For this review, use the dimensioned drawing (mm, ordinates from the lowest corner) and the shaded views. Round coordinates to 2 decimals unless told otherwise and drop trailing zeros. Order: outer loops, then holes, each group sorted by start corner. A loop starts at its lowest first (then second) coordinate and runs counter-clockwise, first axis right, second up. Notation, with made-up numbers: (-29.5, 59) - (4.5, 59) arc R16 cw to (4.5, 70) - close; hole circle Ø6 at (14, -30). An arc over 180 degrees is marked (long way). Write each question's results on one line, items separated by ' | '. Start each with the question number.
(1) Insertion check: pin 1 Ø6 at (x, y) = (13, 81) entering from +Z; pin 2 Ø2 at (x, z) = (41, 4.5) entering from -Y; pin 3 Ø1.9 at (y, z) = (50, 2) entering from +X; pin 4 Ø3 at (y, z) = (67.5, 3) entering from -X. Each pin has a flat end and moves straight along its axis. Give the tip position at first contact, or say it passes through.
(2) For L1, parallel to X at y = 79.5, z = 5; L2, parallel to Y at x = 13, z = 5.75, list the stretches that pass through material, from the lowest coordinate up. Write a range as from..to.
(3) Take a section at A-A, the plane z = 4. Give the boundary of the cut face in (x, y).
(4) Take a section at B-B, the plane x = 7. Give the boundary of the cut face in (y, z).
(5) Take a section at C-C, the plane y = 64.5. Give the boundary of the cut face in (x, z), plus the area to 3 significant figures.
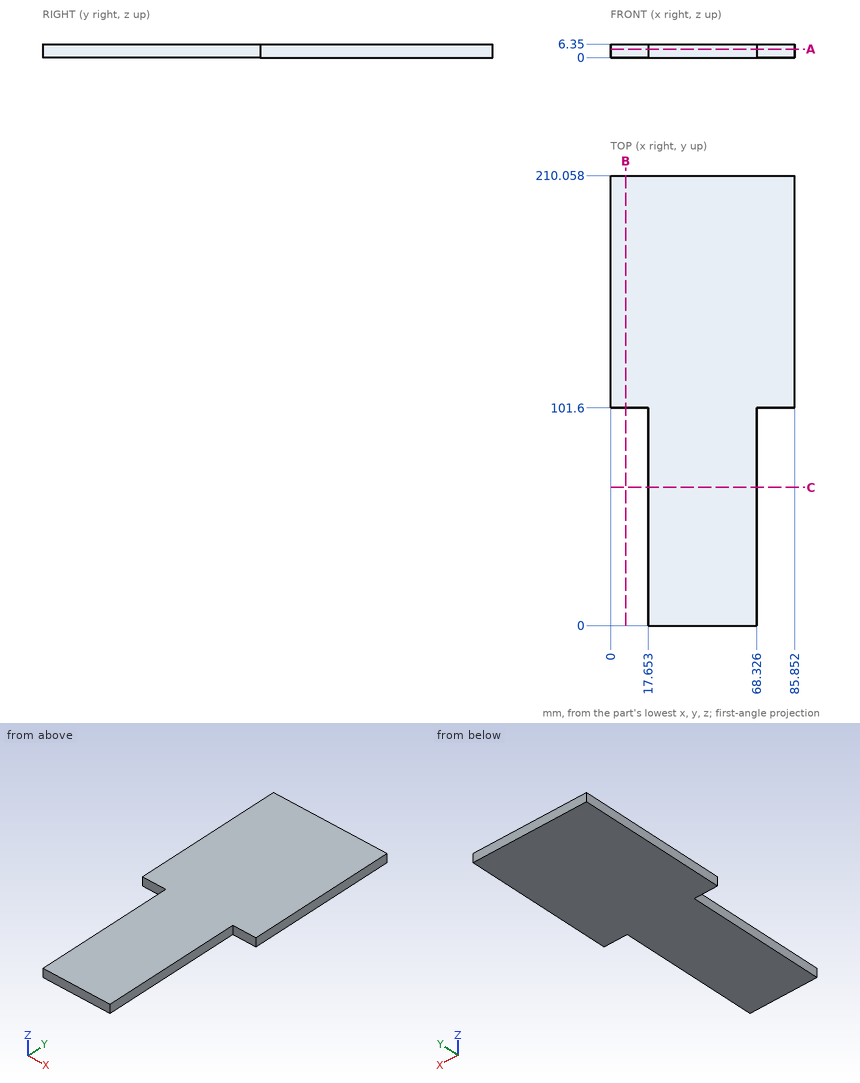
Results below:
1) pin 1: passes through | pin 2: stops at y = 0 | pin 3: stops at x = 68.33 | pin 4: stops at x = 17.65
2) L1: x = 17.65..68.33 | L2: y = 101.6..210.06
3) outline: (0, 101.6) - (17.65, 101.6) - (17.65, 0) - (68.33, 0) - (68.33, 101.6) - (85.85, 101.6) - (85.85, 210.06) - (0, 210.06) - close
4) outline: (101.6, 0) - (210.06, 0) - (210.06, 6.35) - (101.6, 6.35) - close
5) outline: (17.65, 0) - (68.33, 0) - (68.33, 6.35) - (17.65, 6.35) - close | area: 322 mm^2
